```python
from build123d import *

# Parameters (mm, degrees)
CUT_EXTRUDE1_DEPTH      = 47.613731882
CUT_EXTRUDE1_DEPTH_BACK = 47.613731882


with BuildPart() as part:
    # Sketch1 → Revolve1 (revolve)
    with BuildSketch(Plane.XY, mode=Mode.PRIVATE) as revolve1_sk:
        with BuildLine():
            Line((41.2, 10.5), (-10.5, 10.5))
            ThreePointArc((-10.5, 10.5), (-8.266728857, 10.259751459), (-6.135655834, 9.55))
            Line((-6.135655834, 9.55), (42.2, 9.55))
            Line((42.2, 9.55), (42.2, 14))
            Line((42.2, 14), (41.2, 14))
            Line((41.2, 14), (41.2, 10.5))
        make_face()
    revolve(revolve1_sk.sketch.rotate(Axis((0, 0, 0), (1, 0, 0)), 90), axis=Axis((0, 0, 0), (1, 0, 0)))

    # Sketch1_3 → Cut-Extrude1 (cut, two sides: drawn at the far end of the back side and taken through both)
    with BuildSketch(Plane.XY.offset(-CUT_EXTRUDE1_DEPTH_BACK)):
        with BuildLine():
            ThreePointArc((-10.5, -10.5), (-0.240248541, -2.233271143), (-6.135655834, 9.55))
            Line((-6.135655834, 9.55), (-10.5, 9.55))
            Line((-10.5, 9.55), (-10.5, -10.5))
        make_face()
        with BuildLine():
            Line((-10.5, 9.55), (-6.135655834, 9.55))
            ThreePointArc((-6.135655834, 9.55), (-8.266728857, 10.259751459), (-10.5, 10.5))
            Line((-10.5, 10.5), (-10.5, 9.55))
        make_face()
        with BuildLine():
            Line((-10.5, 9.55), (-6.135655834, 9.55))
            ThreePointArc((-6.135655834, 9.55), (-8.266728857, 10.259751459), (-10.5, 10.5))
            Line((-10.5, 10.5), (-10.5, 9.55))
        make_face()
    extrude(amount=CUT_EXTRUDE1_DEPTH + CUT_EXTRUDE1_DEPTH_BACK, mode=Mode.SUBTRACT)


solid = part.part
```
Input: part model. Units: mm. Frame: model coordinates. A direction names the side the tool comes from. Give positions to 0.01 mm unless a question says otherwise; leave off trailing zeros. Order: outer loops, then holes, each group sorted by start corner. A loop starts at its lowest first (then second) coordinate and runs counter-clockwise, first axis right, second up. Notation, with made-up numbers: M -10.75,55.25 L 10.25,55.25 A5 ccw 10.25,62.25 Z; hole C 47.5,-34.5 d8. An arc over 180 degrees is marked long. Return JSON: item names as keys, results as strings.
Item 1: Cut plane A-A (z = 0). Return loops of the section in (x, y), then the cut area to 3 significant figures.
Solutions:
{"outline": "M -10.5,-10.5 L 41.2,-10.5 L 41.2,-14 L 42.2,-14 L 42.2,-9.55 L -6.14,-9.55 A10.5 cw Z; M -10.5,10.5 A10.5 cw -6.14,9.55 L 42.2,9.55 L 42.2,14 L 41.2,14 L 41.2,10.5 Z", "area": "102 mm^2"}
Item 2: Cut plane C-C (x = 3.5). Return loops of the section in (y, z).
Solutions:
{"outline": "C 0,0 d21; hole C 0,0 d19.1"}
Item 3: Cut plane B-B (y = 0). Return loops of the section in (x, z).
Solutions:
{"outline": "M 0,-10.5 L 41.2,-10.5 L 41.2,-14 L 42.2,-14 L 42.2,-9.55 L 0,-9.55 Z; M 0,9.55 L 42.2,9.55 L 42.2,14 L 41.2,14 L 41.2,10.5 L 0,10.5 Z"}
Item 4: Access query for faces 1 (the cylindrical face through (41.7, 12.4, 6.5)), 2 (the flat face through (41.2, -9.4, 5.1)). Directions: +Z, -Z, +X, -X, +Y, -Y. A direction counts if a zero-diameter tool reaches every point of the face in a straight line with its end or side. Return the directions, or none.
Solutions:
{"face 1": "+X, -X", "face 2": "-X"}
Item 5: First-contact query: P1, Ø12, axis at x = 23, z = -8.5, coming from the +Y side; P2, Ø10, axis at x = 32, y = 0.5, coming from the +Z side; P3, Ø10, axis at x = 24, y = -4.5, coming from the -Z side; P4, Ø1, axis at y = -6, z = 6.5, coming from the +X side. Flat tips, straight axial feed; report the tip coordinate or a pass-through.
Solutions:
{"P1": "y = 10.2", "P2": "z = 10.5", "P3": "z = -10.5", "P4": "through"}
Item 6: Ray query, probe 1 along Y at (x, z) = (28.5, 0); probe 2 along X at (y, z) = (12.75, -5.25); probe 3 along Y at (x, z) = (15.5, 1.25). Return the intervals inside material, ascending.
Solutions:
{"probe 1": "-10.5 to -9.55, 9.55 to 10.5", "probe 2": "41.2 to 42.2", "probe 3": "-10.43 to -9.47, 9.47 to 10.43"}
Item 7: Cut plane D-D (y = 12). Return loops of the section in (x, z).
Solutions:
{"outline": "M 41.2,-7.21 L 42.2,-7.21 L 42.2,7.21 L 41.2,7.21 Z"}
Item 8: Pull-direction query (Y, two-part tool) for faces 3 (the flat face through (42.2, 9.14, 3.31)), 4 (the cylindrical face through (20.733, -7.096, -7.739)), 5 (the cylindrical face through (18.37, 3.66, 8.82)); classes: +Y half, -Y half, draft (parallel to the pull), parting line (faces both ways), or undercut.
Solutions:
{"face 3": "draft", "face 4": "parting line", "face 5": "undercut"}
